```python
from build123d import *

# Parameters (mm, degrees)
SKETCH1_W           = 50
SKETCH1_H           = 120
BOSS_EXTRUDE1_DEPTH = 13
FILLET1_R           = 10
SKETCH6_W           = 40
SKETCH6_H           = 110
BOSS_EXTRUDE4_DEPTH = 13
SKETCH7_W           = 40
SKETCH7_H           = 80
BOSS_EXTRUDE5_DEPTH = 26
SKETCH8_R           = 4
BOSS_EXTRUDE6_DEPTH = 13
FILLET4_R           = 10
SKETCH9_W           = 15.181145945
SKETCH9_H           = 7.400808648
BOSS_EXTRUDE7_DEPTH = 0.1


with BuildPart() as part:
    # Sketch1 → Boss-Extrude1 (new body)
    with BuildSketch(Plane(origin=(0, 0, 0), x_dir=(1, 0, 0), z_dir=(0, 1, 0))):
        with Locations((25, 60)):
            Rectangle(SKETCH1_W, SKETCH1_H)
    extrude(amount=BOSS_EXTRUDE1_DEPTH)

    # Fillet1
    fillet1_edges = [part.edges().sort_by_distance(p)[0] for p in [
        (0, 6.5, -120),
        (50, 6.5, -120),
        (50, 6.5, 0),
        (0, 6.5, 0),
    ]]
    fillet(fillet1_edges, radius=FILLET1_R)

    # Sketch6 → Boss-Extrude4 (add)
    with BuildSketch(Plane(origin=(0, 13, 0), x_dir=(1, 0, 0), z_dir=(0, 1, 0))):
        with Locations((25.115018377, 60.006298816)):
            Rectangle(SKETCH6_W, SKETCH6_H)
    extrude(amount=BOSS_EXTRUDE4_DEPTH)

    # Sketch7 → Boss-Extrude5 (add)
    with BuildSketch(Plane(origin=(0, 26, 0), x_dir=(1, 0, 0), z_dir=(0, 1, 0))):
        with Locations((25.115018377, 60.006298816)):
            Rectangle(SKETCH7_W, SKETCH7_H)
    extrude(amount=BOSS_EXTRUDE5_DEPTH)

    # Sketch8 → Boss-Extrude6 (add)
    with BuildSketch(Plane(origin=(0, 26, 0), x_dir=(1, 0, 0), z_dir=(0, 1, 0))):
        with Locations(Location((25.115018377, 107.506298816, 0), (0, 0, 90))):
            Circle(SKETCH8_R)
        with Locations(Location((25.115018377, 12.506298816, 0), (0, 0, 90))):
            Circle(SKETCH8_R)
    extrude(amount=BOSS_EXTRUDE6_DEPTH)

    # Fillet4
    fillet4_edges = [part.edges().sort_by_distance(p)[0] for p in [
        (5.115018377, 19.5, -115.006298816),
        (5.115018377, 19.5, -5.006298816),
        (45.115018377, 19.5, -5.006298816),
        (45.115018377, 19.5, -115.006298816),
        (5.115018377, 39, -100.006298816),
        (5.115018377, 39, -20.006298816),
        (45.115018377, 39, -20.006298816),
        (45.115018377, 39, -100.006298816),
    ]]
    fillet(fillet4_edges, radius=FILLET4_R)

    # Sketch9 → Boss-Extrude7 (add)
    with BuildSketch(Plane(origin=(0, 52, 0), x_dir=(1, 0, 0), z_dir=(0, 1, 0))):
        with Locations((25.189764325, 73.246129728)):
            Rectangle(SKETCH9_W, SKETCH9_H)
        with Locations((25.189764325, 83.246129728)):
            Rectangle(SKETCH9_W, SKETCH9_H)
        with Locations((25.189764325, 63.246129728)):
            Rectangle(SKETCH9_W, SKETCH9_H)
        with Locations((25.189764325, 53.246129728)):
            Rectangle(SKETCH9_W, SKETCH9_H)
        with Locations((25.189764325, 43.246129728)):
            Rectangle(SKETCH9_W, SKETCH9_H)
    extrude(amount=BOSS_EXTRUDE7_DEPTH)


solid = part.part
```
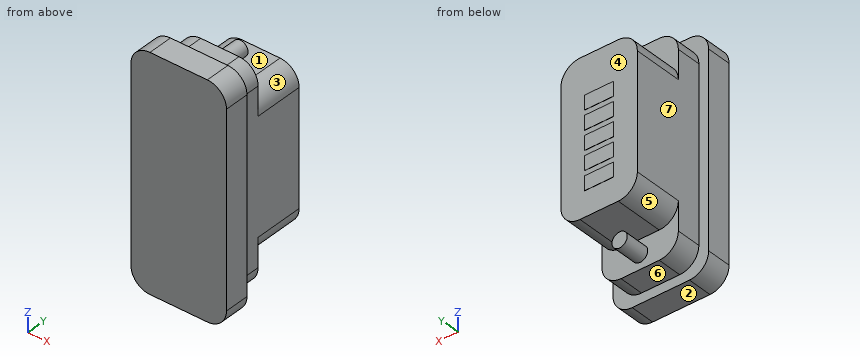
Here's how the part is built. I have some questions about the finished solid (model axes, mm). Face numbers are marked on the shaded views. A direction names the side the tool comes from. Give positions to 0.01 mm unless a question says otherwise; leave off trailing zeros. Order: outer loops, then holes, each group sorted by start corner. A loop starts at its lowest first (then second) coordinate and runs counter-clockwise, first axis right, second up. Notation, with made-up numbers: (-12, 11.25) - (17, 11.25) arc R30 ccw to (17, 35.25) - close; hole circle Ø1 at (34.25, -8.5). An arc over 180 degrees is marked (long way). Answer as a JSON object with one key per item and string values. Group by question number.
Item 1: If we section it at D-D on z = -64: Please give me the cut outline in (x, y).
Item 2: If we section it at C-C on x = 38: Please give me the cut outline in (y, z), and give its area (3 significant figures).
Item 3: If we section it at B-B on z = -35.5: Please give me the cut outline in (x, y), and give its area (3 significant figures).
Item 4: For P1, Ø10, axis at x = 44.5, z = -77, coming from the +Y side; P2, Ø12, axis at x = 36.5, y = 26.5, coming from the -Z side; P3, Ø3, axis at y = 37.5, z = -83, coming from the -X side (3 decimals), each with a flat end and sliding along its axis, tell me the tip position at first contact or that it passes through.
Item 5: Which directions (+Z, -Z, +X, -X, +Y, -Y) give clear straight access to the entire face, cutting with the end or side of a thin tool? Please do the marked faces 4, 5, 6 and 7.
Item 6: Please list where these lines run through material, in increasing order: probe 1 along Z at (x, y) = (34, 19); probe 2 along Y at (x, z) = (13.5, -78); probe 3 along Y at (x, z) = (48.5, -64).
Item 7: If we section it at A-A on y = 20: Please give me the cut outline in (x, z), and give its area (3 significant figures).
Item 8: If we mould it in two halves opening along Z, with no side actions, what happens to the marked faces 1, 2 and 3? For each: pulls with the +Z half, pulls with the -Z half, needs draft (parallel to the pull), parting line crosses it, or undercut.
Result set:
{
 "1": {"outline": "(0, 0) - (50, 0) - (50, 13) - (45.12, 13) - (45.12, 52) - (32.78, 52) - (32.78, 52.1) - (17.6, 52.1) - (17.6, 52) - (5.12, 52) - (5.12, 13) - (0, 13) - close"},
 "2": {"outline": "(0, -120) - (13, -120) - (13, -114.58) - (26, -114.58) - (26, -99.58) - (52, -99.58) - (52, -20.43) - (26, -20.43) - (26, -5.43) - (13, -5.43) - (13, 0) - (0, 0) - close", "area": "5,040 mm²"},
 "3": {"outline": "(0, 0) - (50, 0) - (50, 13) - (45.12, 13) - (45.12, 52) - (5.12, 52) - (5.12, 13) - (0, 13) - close", "area": "2,210 mm²"},
 "4": {"P1": "y = 52", "P2": "z = -115.01", "P3": "x = 5.115"},
 "5": {"face 4": "+Y", "face 5": "-Z, -X, +Y", "face 6": "-Z, +X, -X, +Y", "face 7": "+Z, -Z, -X, +Y"},
 "6": {"probe 1": "-115.01 to -5.01", "probe 2": "0 to 52", "probe 3": "0 to 13"},
 "7": {"outline": "(5.12, -105.01) arc R10 ccw to (15.12, -115.01) - (35.12, -115.01) arc R10 ccw to (45.12, -105.01) - (45.12, -15.01) arc R10 ccw to (35.12, -5.01) - (15.12, -5.01) arc R10 ccw to (5.12, -15.01) - close", "area": "4,310 mm²"},
 "8": {"face 1": "undercut", "face 2": "pulls with the -Z half", "face 3": "pulls with the +Z half"}
}
